Can you work these out from the model? Positions are in its coordinate system, mm. Coordinates: 2 decimals unless noted, no trailing zeros. Loops run counter-clockwise (first coordinate to the right, second up) from the corner with the lowest first, then second, coordinate; pieces in that order, holes last.
Autodesk Inventor part; units mm, degrees
ref_plane "Work Plane3" through (-2.5, 0, 300) normal (0, 0, 1) x (1, 0, 0)
ref_plane "YZ Plane" through (0, 0, 0) normal (1, 0, 0) x (0, 1, 0)
ref_plane "XZ Plane" through (0, 0, 0) normal (0, 1, 0) x (-1, 0, 0)
sketch "Sketch1" plane through (0, 0, 0) normal (0, 0, 1) x (1, 0, 0)
  circle A0 centre (0, 0) radius 2.5
  circle A1 centre (0, 50) radius 2.5
  circle A2 centre (60, 50) radius 2.5
  circle A3 centre (60, 0) radius 2.5
  dimension "d0" = 5
  dimension "d11" = 5
  dimension "d12" = 5
  dimension "d13" = 5
sketch "Sketch2" plane through (0, 0, 0) normal (1, 0, 0) x (0, 1, 0)
  circle A0 centre (0, 0) radius 2.5
  circle A1 centre (50, 0) radius 2.5
  circle A2 centre (0, 300) radius 2.5
  circle A3 centre (50, 300) radius 2.5
  dimension "d1" = 5
  dimension "d27" = 5
  dimension "d35" = 5
  dimension "d36" = 5
sketch "Sketch3" plane through (0, 0, 0) normal (0, 1, 0) x (-1, 0, 0)
  circle A0 centre (0, 0) radius 2.5
  circle A1 centre (-60, 0) radius 2.5
  circle A2 centre (0, 300) radius 2.5
  circle A3 centre (-60, 300) radius 2.5
  dimension "d2" = 5
  dimension "d31" = 5
  dimension "d42" = 5
  dimension "d43" = 5
extrude "LongBL" add sketch "Sketch1" along normal blind 300 contours A0
extrude "SideBB" add sketch "Sketch3" along normal blind 50 contours A0
extrude "UpBL" add sketch "Sketch2" along normal blind 60 contours A0
extrude "LongBR" add sketch "Sketch1" along normal blind 300 contours A3
extrude "LongTL" add sketch "Sketch1" along normal blind 300 contours A1
extrude "LongTR" add sketch "Sketch1" along normal blind 300 contours A2
extrude "Extrusion9" add sketch "Sketch2" along normal blind 60 contours A1
extrude "Extrusion10" add sketch "Sketch3" along normal blind 50 contours A1
extrude "Extrusion11" add sketch "Sketch2" along normal blind 60 contours A3
extrude "Extrusion12" add sketch "Sketch2" along normal blind 60 contours A2
extrude "Extrusion13" add sketch "Sketch3" along normal blind 50 contours A3
extrude "Extrusion14" add sketch "Sketch3" along normal blind 50 contours A2
ref_plane "Work Plane3" through (-2.5, 0, 300) normal (0, 0, 1) x (1, 0, 0)
sketch "Sketch5" plane through (-2.5, 0, 300) normal (0, 0, 1) x (1, 0, 0)
  arc A0 (4.2678, 1.7678) -> (0, 0) centre (2.5, 0) ccw
  line L0 (0, 0) -> (2.5, 0)
  circle A1 centre (2.5, 0) radius 2.5
  line L1 (2.5, 50) -> (2.5, 52.5)
  circle A2 centre (2.5, 50) radius 2.5
  line L2 (62.5, 50) -> (60, 47.5)
  circle A3 centre (62.5, 50) radius 2.5
  arc A4 (60.7322, 1.7678) -> (62.5, -2.5) centre (62.5, 0) ccw
  circle A5 centre (62.5, 0) radius 2.5
  point P0 (60.7322, 48.2322)
  dimension "d48" = 5
  dimension "d49" = 5
  dimension "d50" = 5
  dimension "d51" = 5
extrude "FTLConnect" add sketch "Sketch5" along normal blind 17.5 contours A2
sketch "Sketch7" plane through (-2.5, 0, 300) normal (0, 0, 1) x (1, 0, 0)
  arc A0 (0, 0) -> (2.5, -2.5) centre (2.5, 0) ccw
  line L0 (2.5, -2.5) -> (2.5, 0)
  circle A1 centre (2.5, 0) radius 2.5
  line L1 (65, 50) -> (62.5, 50)
  circle A2 centre (62.5, 50) radius 2.5
  circle A3 centre (62.5, 0) radius 2.5
extrude "FTRConnect" add sketch "Sketch7" along normal blind 17.5 contours A2
sketch "Sketch8" plane through (-2.5, 0, 300) normal (0, 0, 1) x (1, 0, 0)
  line L0 (2.5, -2.5) -> (2.5, 0)
  circle A0 centre (2.5, 0) radius 2.5
  dimension "d56" = 5
extrude "FBLConnect" add sketch "Sketch8" along normal blind 17.5
sketch "Sketch9" plane through (-2.5, 0, 300) normal (0, 0, 1) x (1, 0, 0)
  circle A0 centre (62.5, 0) radius 2.5
  point P0 (2.5, 0)
  dimension "d59" = 5
extrude "FBRConnect" add sketch "Sketch9" along normal blind 17.5
extrude "BTRConnect" add sketch "Sketch1" against normal blind 17.5 contours A2
extrude "BTLConnect" add sketch "Sketch1" against normal blind 17.5 contours A1
extrude "BBRConnect" add sketch "Sketch1" against normal blind 17.5 contours A3
extrude "BBLConnect" add sketch "Sketch1" against normal blind 17.5 contours A0
properties part number "RCPlaneSkeletonModel1" material "PC/ABS Plastic"
(1) I want a section at B-B on x = 29.5. Write out the boundary of the cut face in (y, z).
Check values:
outline: circle Ø5 at (0, 0); circle Ø5 at (0, 300); circle Ø5 at (50, 0); circle Ø5 at (50, 300)
(2) If I drill on probe 1 along Z at (x, y) = (42, 0); probe 2 along Y at (x, z) = (58.5, 125); probe 3 along X at (y, z) = (7.5, 302), over which ranges is the centre line in solid material (lowest first)?
Check values:
probe 1: z = -2.5 to 2.5, 297.5 to 302.5
probe 2: y = -2 to 2, 48 to 52
probe 3: x = -1.5 to 1.5, 58.5 to 61.5
(3) I'm going to push flat-ended pins straight in: pin 1 (3 mm diameter, centred on x = 4.5, z = 80, fed in from +Y); pin 2 (10 mm diameter, centred on x = 5, y = 22, fed in from -Z). Where does each tip first touch, or does it pass through?
Check values:
pin 1: passes through
pin 2: stops at z = -2.5
(4) I want a section at A-A on y = 11. Write out the boundary of the cut face in (x, z).
Check values:
outline: circle Ø5 at (0, 0); circle Ø5 at (0, 300); circle Ø5 at (60, 0); circle Ø5 at (60, 300)
